Geometry check sheet. Reference: the model listing, model coordinates, mm. Coordinates: 2 decimals unless noted, no trailing zeros. Loops run counter-clockwise (first coordinate to the right, second up) from the corner with the lowest first, then second, coordinate; pieces in that order, holes last.
Autodesk Inventor part; units mm, degrees
ref_plane "YZ Plane" through (0, 0, 0) normal (1, 0, 0) x (0, 1, 0)
ref_plane "XZ Plane" through (0, 0, 0) normal (0, 1, 0) x (-1, 0, 0)
ref_plane "XY Plane" through (0, 0, 0) normal (0, 0, 1) x (1, 0, 0)
sketch "Sketch6" plane through (0, 0, 0) normal (0, 0, 1) x (1, 0, 0)
  circle A0 centre (0, 0) radius 3.175
  circle A1 centre (0, 0) radius 19.05
  dimension "d17" = 6.35
  dimension "d18" = 38.1
extrude "Extrusion5" add sketch "Sketch6" along normal blind 381
sketch "Sketch7" plane through (0, 0, 0) normal (1, 0, 0) x (0, 1, 0)
  circle A0 centre (0, 50.8) radius 3.175
  line L0 (19.05, 0) -> (-19.05, 0)
  line L1 (19.05, 0) -> (19.05, 27.0227)
  line L2 (19.05, 0) -> (19.05, 381)
  line L3 (-19.05, 0.4439) -> (-19.05, 5.396)
  line L4 (-19.05, 0) -> (-19.05, 381)
  point P0 (0, 0)
  point P1 (0, 0)
  dimension "d21" = 6.35
  dimension "d22" = 19.05
  dimension "d23" = 19.05
  dimension "d24" = 50.8
extrude "Extrusion6" cut sketch "Sketch7" along normal mid plane 127
properties part number "Shaft connecting chass" material "CFRP"
1) Section check A-A on y = 0. Record the cut outline in (x, z) (3 decimals), and give its area (3 significant figures).
Data:
outline: (-19.05, 0) - (-3.175, 0) - (-3.175, 47.625) - (-19.05, 47.625) - close; (-19.05, 53.975) - (-3.175, 53.975) - (-3.175, 381) - (-19.05, 381) - close; (3.175, 0) - (19.05, 0) - (19.05, 47.625) - (3.175, 47.625) - close; (3.175, 53.975) - (19.05, 53.975) - (19.05, 381) - (3.175, 381) - close
area: 11,900 mm2
2) Mould release check, pull along X, two halves, no side actions. Record for faces 1 (the cylindrical face through (-15.12, 11.59, 187.83)), 2 (the cylindrical face through (-0.69, 3.1, 213.59)), 3 (the flat face through (4, 0, 381)): +X half, -X half, draft (parallel to the pull), parting line (faces both ways), or undercut.
Data:
face 1: parting line
face 2: undercut
face 3: draft
3) Depth check by flat-ended pin: pin 1 (4 mm diameter, centred on y = 0, z = 50.8, fed in from -X); pin 2 (6 mm diameter, centred on x = -2.5, z = 292.5, fed in from -Y); pin 3 (1.5 mm diameter, centred on x = -13, z = 71.5, fed in from -Y); pin 4 (6 mm diameter, centred on y = 8, z = 158.5, fed in from -X). Enter the tip coordinate at first touch or a pass-through.
Data:
pin 1: passes through
pin 2: stops at y = -19.05
pin 3: stops at y = -14.59
pin 4: stops at x = -18.38
4) Section check C-C on z = 257.5. Record the cut outline in (x, y) (3 decimals).
Data:
outline: circle Ø38.1 at (0, 0); hole circle Ø6.35 at (0, 0)
5) Material ranges on probe 1 along Y at (x, z) = (0, 293) (3 decimals); probe 2 along Z at (x, y) = (4, 0) (3 decimals), recorded low to high.
Data:
probe 1: y = -19.05 to -3.175, 3.175 to 19.05
probe 2: z = 0 to 47.625, 53.975 to 381
6) Section check B-B on x = -9. Record the cut outline in (y, z) (3 decimals).
Data:
outline: (-16.79, 0) - (16.79, 0) - (16.79, 381) - (-16.79, 381) - close; hole circle Ø6.35 at (0, 50.8)
